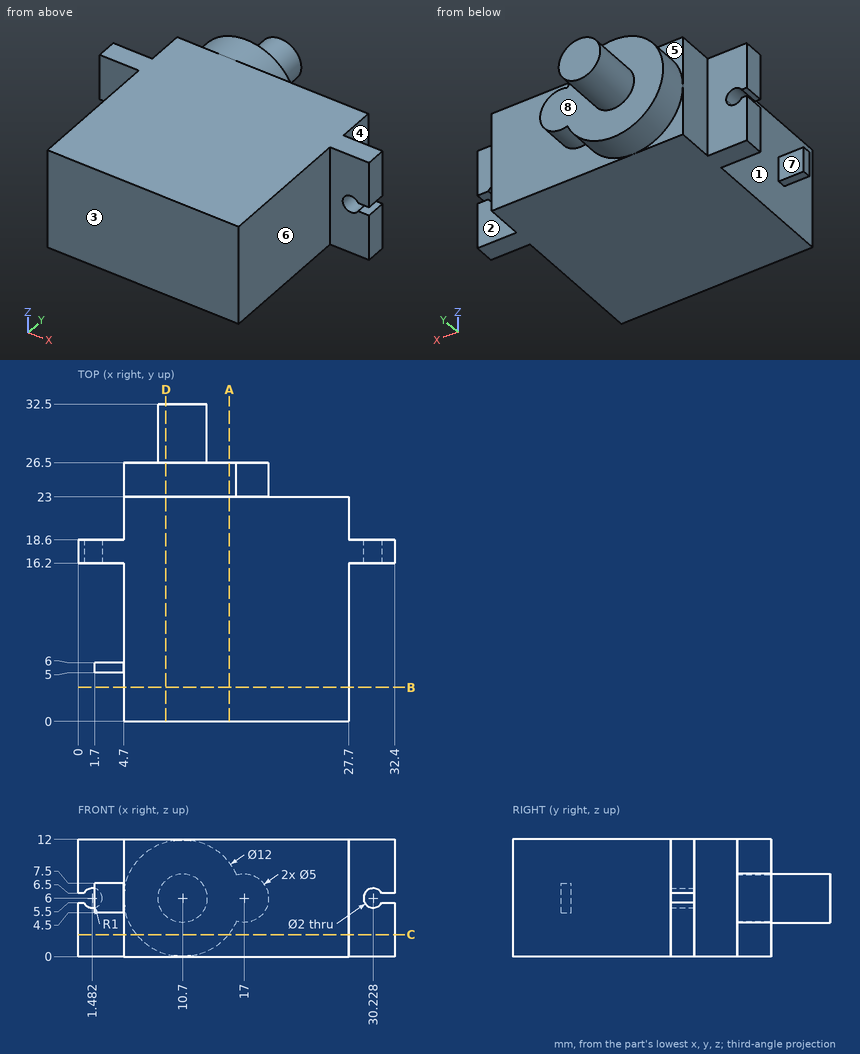
Part print with two shaded views. Sizes in mm from the minimum x, y, z corner. A direction names the side the tool comes from. Give positions to 0.01 mm unless a question says otherwise; leave off trailing zeros. Order: outer loops, then holes, each group sorted by start corner. A loop starts at its lowest first (then second) coordinate and runs counter-clockwise, first axis right, second up.
(1) Tool access for the marked faces 4, 5, 6, 7 and 8: list every direction of +Z, -Z, +X, -X, +Y, -Y with a clear straight run to the whole face (end or side of a thin tool).
(2) Mould opens along Y. For the marked faces 1, 2 and 3 say: released by +Y, released by -Y, zero draft, split by the parting line, or undercut.
(3) Saw through at C-C, the plane z = 2.25. Give the cut face in (x, y), then the cut area to 3 significant figures.
(4) Saw through at A-A, the plane x = 15.5. Give the cut face in (y, z), then the cut area to 3 significant figures.
(5) Drill centre lines: L1, parallel to X at y = 16.8, z = 6; L2, parallel to Y at x = 15.5, z = 6.5; L3, parallel to X at y = 6.5, z = 5.75. Where is each one in solid material? Low to high.
(6) Flat gauge pins, fed straight in: pin 1 (1.5 mm diameter, centred on x = 3.5, z = 6, fed in from +Y); pin 2 (3 mm diameter, centred on x = 30.23, z = 6, fed in from -Y); pin 3 (6 mm diameter, centred on x = 7, y = 28, fed in from -Z). Where does each tip first touch, or does it go through?
(7) Saw through at D-D, the plane x = 9. Give the cut face in (y, z), then the cut area to 3 significant figures.
(8) Saw through at B-B, the plane y = 3.5. Give the cut face in (x, z).
Results found:
1. face 4: +Z, -Z, +X, +Y
1. face 5: +Z, -X, +Y
1. face 6: +Z, -Z, +X, -Y
1. face 7: +Z, -Z, -X
1. face 8: +Y
2. face 1: undercut
2. face 2: released by +Y
2. face 3: released by -Y
3. outline: (0, 16.2) - (4.7, 16.2) - (4.7, 0) - (27.7, 0) - (27.7, 16.2) - (32.4, 16.2) - (32.4, 18.6) - (27.7, 18.6) - (27.7, 23) - (15.38, 23) - (15.38, 26.5) - (6.02, 26.5) - (6.02, 23) - (4.7, 23) - (4.7, 18.6) - (0, 18.6) - close
3. area: 584 mm2
4. outline: (0, 0) - (23, 0) - (23, 2.4) - (26.5, 2.4) - (26.5, 9.6) - (23, 9.6) - (23, 12) - (0, 12) - close
4. area: 301 mm2
5. L1: x = 2.48 to 29.23
5. L2: y = 0 to 26.5
5. L3: x = 4.7 to 27.7
6. pin 1: stops at y = 18.6
6. pin 2: stops at y = 16.2
6. pin 3: stops at z = 0.1
7. outline: (0, 0) - (23, 0) - (23, 0.25) - (26.5, 0.25) - (26.5, 4.17) - (32.5, 4.17) - (32.5, 7.83) - (26.5, 7.83) - (26.5, 11.75) - (23, 11.75) - (23, 12) - (0, 12) - close
7. area: 338 mm2
8. outline: (4.7, 0) - (27.7, 0) - (27.7, 12) - (4.7, 12) - close
